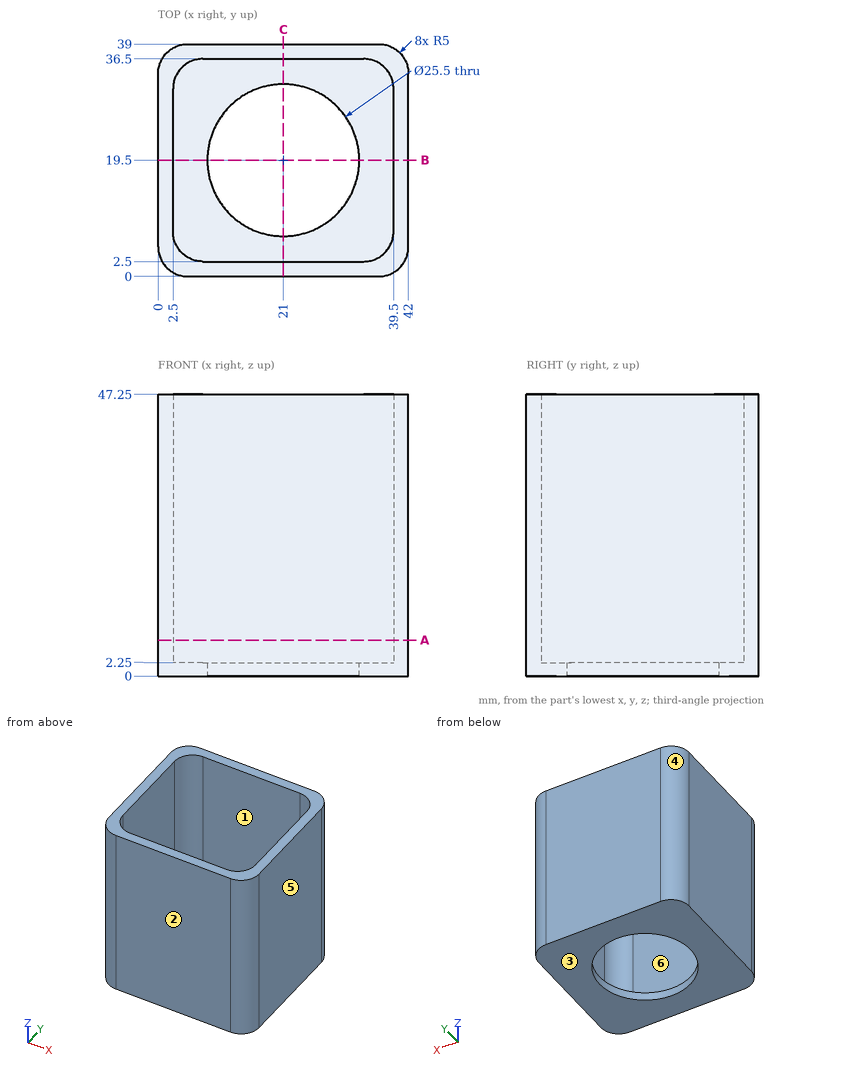
Input: dimensioned drawing with shaded views. Units: mm. Origin: part minimum x, y, z. A direction names the side the tool comes from. Round coordinates to 2 decimals unless told otherwise and drop trailing zeros. Loops run counter-clockwise (first coordinate to the right, second up) from the corner with the lowest first, then second, coordinate; pieces in that order, holes last. Notation, with made-up numbers: (34.25, -29.5) -> (56.25, -29.5) arc R16 cw to (56.25, -8.5) -> close; hole circle Ø1 at (-8, 42). An arc over 180 degrees is marked (long way). One line per item, written item: value.
(1) Pin query (flat end, axial travel): pin 1 (8 mm diameter, centred on x = 30.5, y = 32, fed in from +Z); pin 2 (10 mm diameter, centred on x = 11, z = 22.5, fed in from -Y). Return the tip coordinate at first contact, or that it passes through.
Geometry check:
pin 1: z = 2.25
pin 2: y = 0
(2) Material intervals for line 1 (X direction, y = 23.5, z = 33.5); line 2 (Y direction, x = 17.5, z = 17); line 3 (Y direction, x = 21, z = 1.2), sorted ascending. Write a range as [from, to].
Geometry check:
line 1: [0, 2.5], [39.5, 42]
line 2: [0, 2.5], [36.5, 39]
line 3: [0, 6.75], [32.25, 39]
(3) Section B-B (y = 19.5). Return the cut outline in (x, z).
Geometry check:
outline: (0, 0) -> (8.25, 0) -> (8.25, 2.25) -> (2.5, 2.25) -> (2.5, 47.25) -> (0, 47.25) -> close; (33.75, 0) -> (42, 0) -> (42, 47.25) -> (39.5, 47.25) -> (39.5, 2.25) -> (33.75, 2.25) -> close
(4) Mould query, pull axis X, two halves, no side actions, for the marked faces 3, 4, 5 and 6. Classes: pulls with the +X half, pulls with the -X half, needs draft (parallel to the pull), parting line crosses it, or undercut.
Geometry check:
face 3: needs draft
face 4: pulls with the -X half
face 5: pulls with the +X half
face 6: undercut
(5) Section A-A (z = 6). Return the cut outline in (x, y), plus the area to 3 significant figures.
Geometry check:
outline: (0, 5) arc R5 ccw to (5, 0) -> (37, 0) arc R5 ccw to (42, 5) -> (42, 34) arc R5 ccw to (37, 39) -> (5, 39) arc R5 ccw to (0, 34) -> close; hole (2.5, 7.5) arc R5 ccw to (7.5, 2.5) -> (34.5, 2.5) arc R5 ccw to (39.5, 7.5) -> (39.5, 31.5) arc R5 ccw to (34.5, 36.5) -> (7.5, 36.5) arc R5 ccw to (2.5, 31.5) -> close
area: 380 mm2
(6) Section C-C (x = 21). Return the cut outline in (y, z), plus the area to 3 significant figures.
Geometry check:
outline: (0, 0) -> (6.75, 0) -> (6.75, 2.25) -> (2.5, 2.25) -> (2.5, 47.25) -> (0, 47.25) -> close; (32.25, 0) -> (39, 0) -> (39, 47.25) -> (36.5, 47.25) -> (36.5, 2.25) -> (32.25, 2.25) -> close
area: 255 mm2
(7) Set-up query: the marked faces 1 and 2. Return all of +Z, -Z, +X, -X, +Y, -Y with unobstructed straight access to the full face (end or side cutting, diameter ignored); none if empty.
Geometry check:
face 1: +Z
face 2: +Z, -Z, +X, -X, -Y
